Could you check a few things on this model? Use its own coordinates, in mm. A direction names the side the tool comes from. Give positions to 0.01 mm unless a question says otherwise; leave off trailing zeros. Order: outer loops, then holes, each group sorted by start corner. A loop starts at its lowest first (then second) coordinate and runs counter-clockwise, first axis right, second up.
(1) Will these pins go through, and if not, where does the flat tip stop? pin 1 (2 mm diameter, centred on x = -24.92, z = 19.94, fed in from -Y); pin 2 (2.5 mm diameter, centred on y = 9.5, z = -14.5, fed in from -X).
(2) If we mould it in two halves opening along X, with no side actions, what happens to faces 3 (the flat face through (24, 7, 7.65)), 4 (the flat face through (-24, 12.17, 5)), 5 (the flat face through (28.416, 6, 0))? For each: released by +X, released by -X, zero draft, split by the parting line, or undercut.
(3) Imagine slicing it at A-A, the plane x = -21. Write out the boundary of the cut face in (y, z).
(4) Imagine slicing it at D-D, the plane x = 6. Write out the boundary of the cut face in (y, z), then the cut area to 3 significant figures.
(5) Imagine slicing it at C-C, the plane y = 6. Write out the boundary of the cut face in (x, z).
(6) If I drill on probe 1 along X at (y, z) = (4.75, -17.5); probe 2 along Z at (x, y) = (12, 11.5); probe 3 along X at (y, z) = (11, -20.5), over which ranges is the centre line in solid material (lowest first)?
(7) On a 3-axis mill with a long thin cutter (end or side, diameter ignored), from which of +Z, -Z, +X, -X, +Y, -Y can I reach the whole of each face in a straight line? I mean faces 1 (the flat face through (10, 12.17, -21)), 2 (the flat face through (26, 6.92, 21)). Say none if no direction works.
(8) Imagine slicing it at B-B, the plane y = 11.5. State how many separate pieces and enclosed holes the cut face has, then the cut area to 3 significant figures.
from build123d import *

# Parameters (mm, degrees)
SKETCH1_W              = 56.8325
SKETCH1_H              = 46.9000078
BOSS_EXTRUDE1_DEPTH    = 12.1700036
SKETCH2_W              = 41.2999936
SKETCH2_H              = 40.099996
CUT_EXTRUDE1_DEPTH     = 10.3700072
SKETCH3_W              = 33.3000096
SKETCH3_H              = 32.100012
CUT_EXTRUDE2_DEPTH     = 0.7999984
SKETCH4_W              = 8.1000092
SKETCH4_H              = 10.8000038
CUT_EXTRUDE3_DEPTH     = 3.999992
CUT_EXTRUDE4_START     = -10.3700072
CUT_EXTRUDE4_OUTLINE_W = 6.7650106
CUT_EXTRUDE4_OUTLINE_H = 2.999994
CUT_EXTRUDE4_DEPTH     = 10.3700072
SKETCH6_W              = 6.7650106
SKETCH6_H              = 2.999994
CUT_EXTRUDE5_DEPTH     = 10.3700072
CUT_EXTRUDE6_DEPTH     = 3.999992
CUT_EXTRUDE7_DEPTH     = 5.2500022
SKETCH9_R              = 1.270176684
SKETCH9_R_2            = 1.270176657
CUT_EXTRUDE8_DEPTH     = 38.486962618
CUT_EXTRUDE10_DEPTH    = 2.3114
CUT_EXTRUDE11_DEPTH    = 0.4886198
CUT_EXTRUDE12_DEPTH    = 7.4324972
SKETCH14_W             = 2.5908
SKETCH14_H             = 5.8999882
CUT_EXTRUDE13_DEPTH    = 1.7031716
CUT_EXTRUDE15_DEPTH    = 2.5908


# Read off the part's stored shape, not the designer's step: Cut-Extrude4
with BuildPart() as part:
    # Sketch1 → Boss-Extrude1 (new body)
    with BuildSketch(Plane(origin=(0, 0, 0), x_dir=(1, 0, 0), z_dir=(0, 1, 0))):
        Rectangle(SKETCH1_W, SKETCH1_H)
    extrude(amount=BOSS_EXTRUDE1_DEPTH)

    # Sketch2 → Cut-Extrude1 (cut)
    with BuildSketch(Plane(origin=(0, 12.1700036, 0), x_dir=(1, 0, 0), z_dir=(0, 1, 0))):
        with Locations((0.333756, 0.5999861)):
            Rectangle(SKETCH2_W, SKETCH2_H)
    extrude(amount=-CUT_EXTRUDE1_DEPTH, mode=Mode.SUBTRACT)

    # Sketch3 → Cut-Extrude2 (cut)
    with BuildSketch(Plane(origin=(0, 1.7999964, 0), x_dir=(1, 0, 0), z_dir=(0, 1, 0))):
        with Locations((0.345948, 0.6121781)):
            Rectangle(SKETCH3_W, SKETCH3_H)
    extrude(amount=-CUT_EXTRUDE2_DEPTH, mode=Mode.SUBTRACT)

    # Sketch4 → Cut-Extrude3 (cut)
    with BuildSketch(Plane(origin=(0, 12.1700036, 0), x_dir=(1, 0, 0), z_dir=(0, 1, 0))):
        with Locations((-24.3662454, 18.050002)):
            Rectangle(SKETCH4_W, SKETCH4_H)
    extrude(amount=-CUT_EXTRUDE3_DEPTH, mode=Mode.SUBTRACT)

    # Cut-Extrude4 outline → Cut-Extrude4 (cut)
    with BuildSketch(Plane(origin=(0, 12.1700036, 0), x_dir=(1, 0, 0), z_dir=(0, 1, 0)).offset(CUT_EXTRUDE4_START)):
        with Locations((-23.6987461, -9.1500071)):
            Rectangle(CUT_EXTRUDE4_OUTLINE_W, CUT_EXTRUDE4_OUTLINE_H)
    extrude(amount=CUT_EXTRUDE4_DEPTH, mode=Mode.SUBTRACT)

    # Sketch6 → Cut-Extrude5 (cut)
    with BuildSketch(Plane(origin=(0, 12.1700036, 0), x_dir=(1, 0, 0), z_dir=(0, 1, 0))):
        with Locations((24.3662581, -9.1500071)):
            Rectangle(SKETCH6_W, SKETCH6_H)
    extrude(amount=-CUT_EXTRUDE5_DEPTH, mode=Mode.SUBTRACT)

    # Sketch7 → Cut-Extrude6 (cut)
    with BuildSketch(Plane.XY.offset(23.4500039)):
        with BuildLine():
            Line((-3.3462468, 12.1700036), (-16.946245, 12.1700036))
            ThreePointArc((-16.946245, 12.1700036), (-10.1462459, 5.3699918), (-3.3462468, 12.1700036))
        make_face()
    extrude(amount=-CUT_EXTRUDE6_DEPTH, mode=Mode.SUBTRACT)

    # Sketch8 → Cut-Extrude7 (cut)
    with BuildSketch(Plane(origin=(0, 12.1700036, 0), x_dir=(1, 0, 0), z_dir=(0, 1, 0))):
        Polygon((-24.916257, -18.0069617), (-26.591255007, -18.97402225), (-26.591255007, -20.90814335), (-24.916257, -21.8752039), (-23.241258993, -20.90814335), (-23.241258993, -18.97402225), align=None)
        Polygon((-24.916257, 11.0930309), (-26.591255007, 10.12597035), (-26.591255007, 8.19184925), (-24.916257, 7.2247887), (-23.241258993, 8.19184925), (-23.241258993, 10.12597035), align=None)
        Polygon((24.9162316, 21.8930347), (23.241233593, 20.92597415), (23.241233593, 18.99185305), (24.9162316, 18.0247925), (26.591229607, 18.99185305), (26.591229607, 20.92597415), align=None)
        Polygon((24.9162316, -18.0069617), (23.241233593, -18.97402225), (23.241233593, -20.90814335), (24.9162316, -21.8752039), (26.591229607, -20.90814335), (26.591229607, -18.97402225), align=None)
    extrude(amount=-CUT_EXTRUDE7_DEPTH, mode=Mode.SUBTRACT)

    # Sketch9 → Cut-Extrude8 (cut, through all)
    with BuildSketch(Plane(origin=(0, 6.9200014, 0), x_dir=(1, 0, 0), z_dir=(0, 1, 0))):
        with Locations(Location((-24.875109, 9.1588971, 0), (0, 0, 270))):
            Circle(SKETCH9_R)
        with Locations(Location((-24.916257, -19.9410828, 0), (0, 0, 270))):
            Circle(SKETCH9_R_2)
        with Locations(Location((24.9162316, -19.9410828, 0), (0, 0, 270))):
            Circle(SKETCH9_R_2)
        with Locations(Location((24.9162316, 19.9589136, 0), (0, 0, 270))):
            Circle(SKETCH9_R_2)
    extrude(amount=-CUT_EXTRUDE8_DEPTH, mode=Mode.SUBTRACT)

    # Sketch11 → Cut-Extrude10 (cut)
    with BuildSketch(Plane.XY.offset(-20.6499841)):
        Polygon((-13.093837264, 10.4681909), (-10.1462332, 8.7663909), (-7.198629136, 10.4681909), (-7.198629136, 13.8717909), (-10.1462332, 15.5735909), (-13.093837264, 13.8717909), align=None)
    extrude(amount=-CUT_EXTRUDE10_DEPTH, mode=Mode.SUBTRACT)

    # Sketch12 → Cut-Extrude11 (cut)
    with BuildSketch(Plane.XY.offset(-22.9613841)):
        with BuildLine():
            ThreePointArc((-8.3962367, 12.1700036), (-10.1462332, 13.9200001), (-11.8962297, 12.1700036))
            Line((-11.8962297, 12.1700036), (-8.3962367, 12.1700036))
        make_face()
        with BuildLine():
            Line((-8.3962367, 12.1700036), (-11.8962297, 12.1700036))
            ThreePointArc((-11.8962297, 12.1700036), (-10.1462332, 10.4200071), (-8.3962367, 12.1700036))
        make_face()
    extrude(amount=-CUT_EXTRUDE11_DEPTH, mode=Mode.SUBTRACT)

    # Sketch13 → Cut-Extrude12 (cut)
    with BuildSketch(Plane(origin=(28.41625, 0, 0), x_dir=(0, 0, -1), z_dir=(1, 0, 0))):
        with BuildLine():
            ThreePointArc((16.1999803, 12.1700036), (14.4499838, 13.9200001), (12.6999873, 12.1700036))
            Line((12.6999873, 12.1700036), (16.1999803, 12.1700036))
        make_face()
        with BuildLine():
            Line((16.1999803, 12.1700036), (12.6999873, 12.1700036))
            ThreePointArc((12.6999873, 12.1700036), (14.4499838, 10.4200071), (16.1999803, 12.1700036))
        make_face()
        with BuildLine():
            Line((-16.2000057, 12.1700036), (-12.7000127, 12.1700036))
            ThreePointArc((-12.7000127, 12.1700036), (-14.4500092, 13.9200001), (-16.2000057, 12.1700036))
        make_face()
        with BuildLine():
            ThreePointArc((-16.2000057, 12.1700036), (-14.4500092, 10.4200071), (-12.7000127, 12.1700036))
            Line((-12.7000127, 12.1700036), (-16.2000057, 12.1700036))
        make_face()
    extrude(amount=-CUT_EXTRUDE12_DEPTH, mode=Mode.SUBTRACT)

    # Sketch14 → Cut-Extrude13 (cut)
    with BuildSketch(Plane(origin=(0, 12.1700036, 0), x_dir=(1, 0, 0), z_dir=(0, 1, 0))):
        with Locations((26.120852, -14.4500092)):
            Rectangle(SKETCH14_W, SKETCH14_H)
    extrude(amount=-CUT_EXTRUDE13_DEPTH, mode=Mode.SUBTRACT)

    # Sketch16 → Cut-Extrude15 (cut)
    with BuildSketch(Plane.ZY.offset(-27.416252)):
        with BuildLine():
            Line((14.4500092, 8.763635), (17.4000033, 10.466832))
            Line((17.4000033, 10.466832), (14.852121437, 10.466832))
            ThreePointArc((14.852121437, 10.466832), (15.822266967, 11.084003429), (16.2000057, 12.1700036))
            Line((16.2000057, 12.1700036), (11.5000151, 12.1700036))
            Line((11.5000151, 12.1700036), (11.5000151, 10.466832))
            Line((11.5000151, 10.466832), (14.4500092, 8.763635))
        make_face()
        Polygon((-17.3999779, 12.1700036), (-17.3999779, 10.466832), (-14.4499838, 8.763635), (-11.4999897, 10.466832), (-11.4999897, 12.1700036), align=None)
    extrude(amount=CUT_EXTRUDE15_DEPTH, mode=Mode.SUBTRACT)


solid = part.part
Answer block:
1. pin 1: passes through
1. pin 2: stops at x = 20.98
2. face 3: undercut
2. face 4: zero draft
2. face 5: released by +X
3. outline: (0, -23.45) - (8.17, -23.45) - (8.17, -12.65) - (12.17, -12.65) - (12.17, 7.65) - (1.8, 7.65) - (1.8, 10.65) - (12.17, 10.65) - (12.17, 23.45) - (0, 23.45) - close
4. outline: (0, -23.45) - (12.17, -23.45) - (12.17, -20.65) - (1.8, -20.65) - (1.8, -16.66) - (1, -16.66) - (1, 15.44) - (1.8, 15.44) - (1.8, 19.45) - (12.17, 19.45) - (12.17, 23.45) - (0, 23.45) - close
4. area: 129 mm2
5. outline: (-28.42, -23.45) - (28.42, -23.45) - (28.42, 23.45) - (-7.29, 23.45) - (-7.29, 19.45) - (20.98, 19.45) - (20.98, 10.65) - (27.75, 10.65) - (27.75, 7.65) - (20.98, 7.65) - (20.98, -20.65) - (-20.32, -20.65) - (-20.32, 7.65) - (-27.08, 7.65) - (-27.08, 10.65) - (-20.32, 10.65) - (-20.32, 19.45) - (-13, 19.45) - (-13, 23.45) - (-28.42, 23.45) - close; hole circle Ø2.54 at (-24.92, 19.94); hole circle Ø2.54 at (-24.88, -9.16); hole circle Ø2.54 at (24.92, -19.96); hole circle Ø2.54 at (24.92, 19.94)
6. probe 1: x = -28.42 to -20.32, 20.98 to 28.42
6. probe 2: z = -23.45 to -20.65, 19.45 to 23.45
6. probe 3: x = 20.98 to 23.24, 26.59 to 28.42
7. face 1: +Z, -Z, +X, -X, +Y
7. face 2: +Y
8. separate pieces: 5
8. enclosed holes: 4
8. area: 711 mm2
